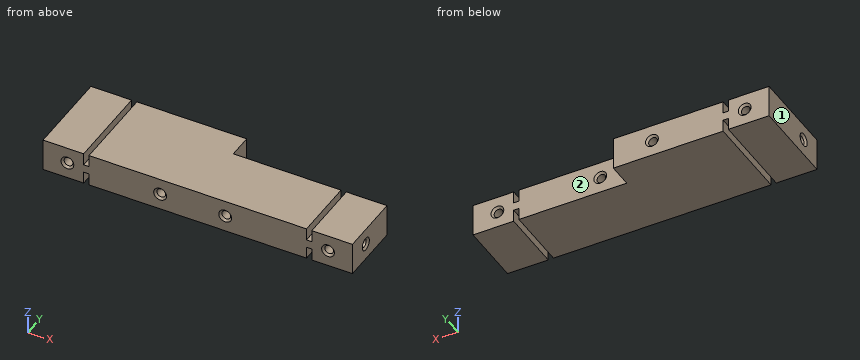
from build123d import *

# Parameters (mm, degrees)
PAD_DEPTH       = 16
SKETCH001_R     = 2.15
SKETCH001_W     = 2.6
SKETCH001_H     = 6
POCKET_DEPTH    = 43.001
CHAMFER_SIZE    = 1
SKETCH002_R     = 2.15
POCKET001_DEPTH = 8
SKETCH003_R     = 2.15
POCKET002_DEPTH = 8
CHAMFER001_SIZE = 1


with BuildPart() as part:
    # Sketch → Pad (new body)
    with BuildSketch(Plane.XY):
        Polygon((0, 0), (0, 43), (76.6, 43), (76.6, 31), (152.2, 31), (152.2, 0), align=None)
    extrude(amount=PAD_DEPTH)

    # Sketch001 → Pocket (cut, through all)
    with BuildSketch(Plane.XZ):
        with Locations((12, 8)):
            Circle(SKETCH001_R)
        with Locations((89.6, 8)):
            Circle(SKETCH001_R)
        with Locations((140.2, 8)):
            Circle(SKETCH001_R)
        with Locations((57.6, 8)):
            Circle(SKETCH001_R)
        with Locations((21.3, 3)):
            Rectangle(SKETCH001_W, SKETCH001_H)
        with Locations((21.3, 13)):
            Rectangle(SKETCH001_W, SKETCH001_H)
        with Locations((130.9, 13)):
            Rectangle(SKETCH001_W, SKETCH001_H)
        with Locations((130.9, 3)):
            Rectangle(SKETCH001_W, SKETCH001_H)
    extrude(amount=-POCKET_DEPTH, mode=Mode.SUBTRACT)

    # Chamfer
    chamfer_edges = [part.edges().sort_by_distance(p)[0] for p in [
        (9.85, 0, 8),
        (55.45, 0, 8),
        (87.45, 0, 8),
        (138.05, 0, 8),
        (9.85, 43, 8),
        (55.45, 43, 8),
        (87.45, 31, 8),
        (138.05, 31, 8),
    ]]
    chamfer(chamfer_edges, length=CHAMFER_SIZE)

    # Sketch002 → Pocket001 (cut)
    with BuildSketch(Plane.YZ):
        with Locations((12, 8)):
            Circle(SKETCH002_R)
    extrude(amount=POCKET001_DEPTH, mode=Mode.SUBTRACT)

    # Sketch003 (on DatumPlane) → Pocket002 (cut)
    with BuildSketch(Plane.YZ.offset(152.2)):
        with Locations((12, 8)):
            Circle(SKETCH003_R)
    extrude(amount=-POCKET002_DEPTH, mode=Mode.SUBTRACT)

    # Chamfer001
    chamfer001_edges = [part.edges().sort_by_distance(p)[0] for p in [
        (152.2, 9.85, 8),
        (0, 9.85, 8),
    ]]
    chamfer(chamfer001_edges, length=CHAMFER001_SIZE)


solid = part.part
For this review, take the finished solid that the model builds, in its own axes (mm). Face numbers are marked on the shaded views. A direction names the side the tool comes from. Round coordinates to 2 decimals unless told otherwise and drop trailing zeros. Loops run counter-clockwise (first coordinate to the right, second up) from the corner with the lowest first, then second, coordinate; pieces in that order, holes last. Notation, with made-up numbers: (22.5, 51) - (80.5, 51) arc R5 ccw to (80.5, 55) - close; hole circle Ø11 at (30.25, 28.25). An arc over 180 degrees is marked (long way). Answer as CSV lines item,"result".
(1) Wall thickness on line 1 (X direction, y = 14.5, z = 12.75); line 2 (X direction, y = 25.5, z = 7.25); line 3 (Z direction, x = 140, y = 13): over which ranges is each line inside the solid? List them lowest first.
Checked values:
line 1,"x = 0 to 20, 22.6 to 129.6, 132.2 to 152.2"
line 2,"x = 0 to 9.99, 14.01 to 55.59, 59.61 to 87.59, 91.61 to 138.19, 142.21 to 152.2"
line 3,"z = 0 to 5.86, 10.14 to 16"
(2) Insertion check: P1, Ø3.5, axis at y = 12, z = 8, coming from the -X side; P2, Ø6, axis at x = 18, y = 24.5, coming from the -Z side; P3, Ø4.5, axis at y = 11.5, z = 8, coming from the -X side; P4, Ø5, axis at x = 140.2, z = 8, coming from the +Y side. Each pin has a flat end and moves straight along its axis. Give the tip position at first contact, or say it passes through.
Checked values:
P1,"stops at x = 8"
P2,"stops at z = 0"
P3,"stops at x = 0.4"
P4,"stops at y = 30.35"
(3) Consider section A-A on y = 37. Give the boundary of the cut face in (x, z).
Checked values:
outline,"(0, 0) - (20, 0) - (20, 6) - (22.6, 6) - (22.6, 0) - (76.6, 0) - (76.6, 16) - (22.6, 16) - (22.6, 10) - (20, 10) - (20, 16) - (0, 16) - close; hole circle Ø4.3 at (12, 8); hole circle Ø4.3 at (57.6, 8)"
(4) Tool access review of the marked faces 1 and 2: name each direction out of +Z, -Z, +X, -X, +Y, -Y from which nothing blocks a thin tool from reaching the whole face with its end or side.
Checked values:
face 1,"+Z, -Z, -X, +Y, -Y"
face 2,"+Z, -Z, +X, +Y"
(5) Consider section D-D on y = 27.5. Give the boundary of the cut face in (x, z).
Checked values:
outline,"(0, 0) - (20, 0) - (20, 6) - (22.6, 6) - (22.6, 0) - (129.6, 0) - (129.6, 6) - (132.2, 6) - (132.2, 0) - (152.2, 0) - (152.2, 16) - (132.2, 16) - (132.2, 10) - (129.6, 10) - (129.6, 16) - (22.6, 16) - (22.6, 10) - (20, 10) - (20, 16) - (0, 16) - close; hole circle Ø4.3 at (12, 8); hole circle Ø4.3 at (57.6, 8); hole circle Ø4.3 at (89.6, 8); hole circle Ø4.3 at (140.2, 8)"
(6) Consider section B-B on x = 89.6. Give the boundary of the cut face in (y, z).
Checked values:
outline,"(0, 0) - (31, 0) - (31, 4.85) - (30, 5.85) - (1, 5.85) - (0, 4.85) - close; (0, 11.15) - (1, 10.15) - (30, 10.15) - (31, 11.15) - (31, 16) - (0, 16) - close"
(7) Consider section C-C on z = 14.5. Give the boundary of the cut face in (x, y).
Checked values:
outline,"(0, 0) - (20, 0) - (20, 43) - (0, 43) - close; (22.6, 0) - (129.6, 0) - (129.6, 31) - (76.6, 31) - (76.6, 43) - (22.6, 43) - close; (132.2, 0) - (152.2, 0) - (152.2, 31) - (132.2, 31) - close"
